The listing builds one solid part. Answer for the finished solid, in the listing's coordinates (mm). Give positions to 0.01 mm unless a question says otherwise; leave off trailing zeros. Order: outer loops, then holes, each group sorted by start corner. A loop starts at its lowest first (then second) coordinate and runs counter-clockwise, first axis right, second up. Notation, with made-up numbers: (82.25, 18) - (116.25, 18) arc R12 cw to (116.25, 26) - close; hole circle Ø6 at (-3.5, 65). An arc over 180 degrees is marked (long way). Write each question's results on one line, items separated by ' | '. Start each with the question number.
1. Section C-C (y = 9.5) is taken. Give the vertices of the cut face in (x, z).
2. Find the intervals of material crossed by L1, parallel to X at y = 16.5, z = -178; L2, parallel to Y at x = -1, z = -98 (3 decimals); L3, parallel to X at y = 5.25, z = -125.5, in increasing order.
3. Section B-B (z = -122.5) is taken. Give the vertices of the cut face in (x, y) (1 decimal), and give its area (3 significant figures).
4. Section A-A (x = -5.75) is taken. Give the vertices of the cut face in (y, z) (3 decimals), and give its area (3 significant figures).
5. Flat-ended cylindrical pins translate along their axes: pin 1 (2 mm diameter, centred on x = -6, z = -172.5, fed in from -Y); pin 2 (6 mm diameter, centred on x = -7, y = 14, fed in from -Z); pin 3 (1.7 mm diameter, centred on x = -0.5, z = -127.5, fed in from -Y). Find the tip coordinate at first contact, or state that the pin passes through.
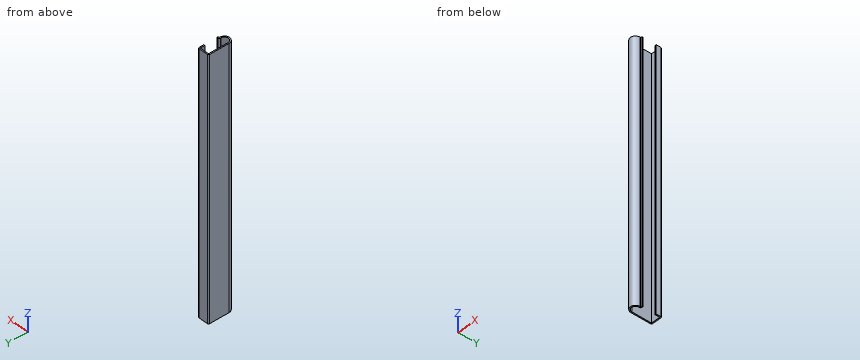
from build123d import *

# Parameters (mm, degrees)
EXTRUDE_THIN1_DEPTH = 285.75
FILLET1_R           = 1.27


with BuildPart() as part:
    # Sketch1 → Extrude-Thin1 (new body)
    with BuildSketch(Plane.XY):
        with BuildLine():
            Line((0, 0), (-1.5875, 0))
            Line((-1.5875, 0), (-1.5875, -0.79375))
            ThreePointArc((-1.5875, -0.79375), (-7.14375, -6.35), (-12.7, -0.79375))
            Line((-12.7, -0.79375), (-12.7, 22.225))
            Line((-12.7, 22.225), (0, 22.225))
            Line((0, 22.225), (0, 15.875))
            Line((0, 15.875), (-1.27, 15.875))
            Line((-1.27, 15.875), (-1.27, 20.955))
            Line((-1.27, 20.955), (-11.43, 20.955))
            Line((-11.43, 20.955), (-11.43, -0.79375))
            ThreePointArc((-11.43, -0.79375), (-7.14375, -5.08), (-2.8575, -0.79375))
            Line((-2.8575, -0.79375), (-2.8575, 1.27))
            Line((-2.8575, 1.27), (0, 1.27))
            Line((0, 1.27), (0, 0))
        make_face()
    extrude(amount=-EXTRUDE_THIN1_DEPTH)

    # Fillet1
    fillet1_edges = [part.edges().sort_by_distance(p)[0] for p in [
        (-2.8575, 1.27, -142.875),
        (-12.7, 22.225, -142.875),
        (0, 22.225, -142.875),
    ]]
    fillet(fillet1_edges, radius=FILLET1_R)


solid = part.part
Reported:
1) outline: (-12.7, -285.75) - (-11.43, -285.75) - (-11.43, 0) - (-12.7, 0) - close
2) L1: -12.7 to -11.43, -1.27 to 0 | L2: 0 to 1.27, 15.875 to 22.196 | L3: -12.7 to -11.43
3) outline: (-12.7, -0.8) arc R5.6 ccw to (-1.6, -0.8) - (-1.6, 0) - (0, 0) - (0, 1.3) - (-1.6, 1.3) arc R1.3 ccw to (-2.9, 0) - (-2.9, -0.8) arc R4.3 cw to (-11.4, -0.8) - (-11.4, 21) - (-1.3, 21) - (-1.3, 15.9) - (0, 15.9) - (0, 21) arc R1.3 ccw to (-1.3, 22.2) - (-11.4, 22.2) arc R1.3 ccw to (-12.7, 21) - close | area: 73.4 mm²
4) outline: (-6.172, -285.75) - (-4.847, -285.75) - (-4.847, 0) - (-6.172, 0) - close; (20.955, -285.75) - (22.225, -285.75) - (22.225, 0) - (20.955, 0) - close | area: 742 mm²
5) pin 1: y = -6.35 | pin 2: through | pin 3: y = 0
